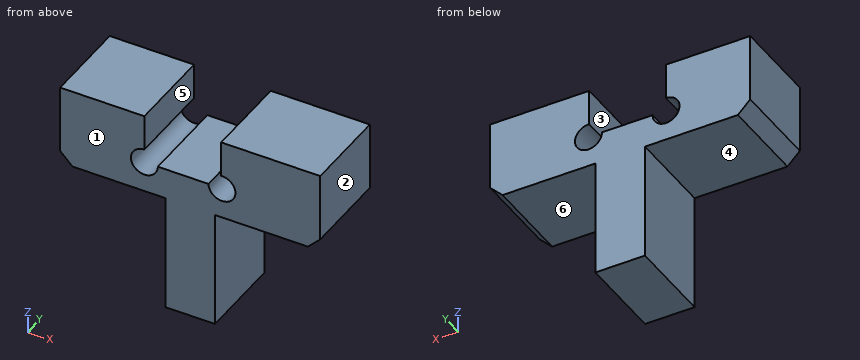
from build123d import *

# Parameters (mm, degrees)
BOSS_EXTRUDE1_DEPTH = 3.5
CHAMFER1_SIZE       = 0.5


with BuildPart() as part:
    # Sketch1 → Boss-Extrude1 (new body)
    with BuildSketch(Plane(origin=(0, 0, 0), x_dir=(1, 0, 0), z_dir=(0, 1, 0))):
        with BuildLine():
            Line((-5.25, -0.51424544), (-1.85, -0.51424544))
            Line((-1.85, -0.51424544), (-1.85, 0.942004129))
            ThreePointArc((-1.85, 0.942004129), (-2.234489618, 1.870244178), (-1.306249568, 1.48575456))
            Line((-1.306249568, 1.48575456), (0.738401898, 1.48575456))
            ThreePointArc((0.738401898, 1.48575456), (1.677846262, 1.85870341), (1.25, 0.942955555))
            Line((1.25, 0.942955555), (1.25, -0.51424544))
            Line((1.25, -0.51424544), (5.25, -0.51424544))
            Line((5.25, -0.51424544), (5.25, 2.74500456))
            Line((5.25, 2.74500456), (1, 2.74500456))
            Line((1, 2.74500456), (1, 7.49500456))
            Line((1, 7.49500456), (-1, 7.49500456))
            Line((-1, 7.49500456), (-1, 2.74500456))
            Line((-1, 2.74500456), (-5.25, 2.74500456))
            Line((-5.25, 2.74500456), (-5.25, -0.51424544))
        make_face()
    extrude(amount=BOSS_EXTRUDE1_DEPTH)

    # Chamfer1
    chamfer1_edges = [part.edges().sort_by_distance(p)[0] for p in [
        (5.25, 1.75, -2.74500456),
        (-5.25, 1.75, -2.74500456),
    ]]
    chamfer(chamfer1_edges, length=CHAMFER1_SIZE)


solid = part.part
The listing builds one solid part. Answer for the finished solid, in the listing's coordinates (mm). Face numbers are marked on the shaded views. A direction names the side the tool comes from. Coordinates: 2 decimals unless noted, no trailing zeros. Write each loop counter-clockwise with the first axis right and the second up, starting at its lowest first coordinate (ties: lowest second). Pieces come first, ordered by that corner, then holes. Notation, with made-up numbers: (10.5, 19.5) -> (58.5, 19.5) arc R8 ccw to (58.5, 25.5) -> close; hole circle Ø7 at (72, -30). An arc over 180 degrees is marked (long way). One line per question, with ' | ' between items.
1. Section A-A (z = -0.5) is taken. Determine the outline of the cut face in (x, y), and give its area (3 significant figures).
Verdict:
outline: (-5.25, 0) -> (-1.85, 0) -> (-1.85, 3.5) -> (-5.25, 3.5) -> close; (1.25, 0) -> (5.25, 0) -> (5.25, 3.5) -> (1.25, 3.5) -> close | area: 25.9 mm^2
2. Section D-D (z = -6.75) is taken. Determine the outline of the cut face in (x, y).
Verdict:
outline: (-1, 0) -> (1, 0) -> (1, 3.5) -> (-1, 3.5) -> close
3. Straight lines are drawn through the part: line 1 (X direction, y = 0.9, z = -0.25); line 2 (X direction, y = 3.05, z = -3.5); line 3 (Z direction, x = 1.5, y = 1.6) (3 decimals). For each, find the intervals that lie inside material, in ascending order.
Verdict:
line 1: x = -5.25 to -1.85, 1.25 to 5.25 | line 2: x = -1 to 1 | line 3: z = -2.745 to -1.984, -0.988 to 0.514
4. Given pin 1 Ø1 at (x, y) = (-0.5, 1) entering from +Z; pin 2 Ø1 at (y, z) = (2, -4) entering from -X, each flat-ended and moving along its own axis, determine where each tip first touches the part or whether it passes through.
Verdict:
pin 1: stops at z = -1.49 | pin 2: stops at x = -1
5. Section C-C (x = 0.5) is taken. Determine the outline of the cut face in (y, z) (3 decimals), and give its area (3 significant figures).
Verdict:
outline: (0, -7.495) -> (3.5, -7.495) -> (3.5, -1.486) -> (0, -1.486) -> close | area: 21.0 mm^2
6. For a pull along X with two mould halves and no side action, classify the marked faces 1, 2 and 3 as released by +X, released by -X, zero draft, split by the parting line, or undercut.
Verdict:
face 1: zero draft | face 2: released by +X | face 3: undercut
7. Which of the six approach directions +Z, -Z, +X, -X, +Y, -Y give full straight-line access (tool end or side, diameter ignored) to the marked faces 4, 5 and 6?
Verdict:
face 4: -Z, -X, +Y, -Y | face 5: +Z, +Y, -Y | face 6: -Z, +X, +Y, -Y
